Could you check a few things on this model? Use its own coordinates, in mm. Face numbers are marked on the shaded views. A direction names the side the tool comes from. Give positions to 0.01 mm unless a question says otherwise; leave off trailing zeros. Loops run counter-clockwise (first coordinate to the right, second up) from the corner with the lowest first, then second, coordinate; pieces in that order, holes last.
1. Imagine slicing it at A-A (z = 14.5). List the corners of the cut face in (x, y) for me, plus the area to 3 significant figures.
2. Thinking about a two-plate mould opening in Z: for the marked faces 3, 4 and 5, which applies, +Z half, -Z half, draft (parallel to the pull), parting line (faces both ways), or undercut?
3. I need wall thicknesses on line 1 along X through (y, z) = (-11, 15); line 2 along Z through (x, y) = (-6.5, 0.5); line 3 along Z through (x, y) = (23, 0.5). Which ranges of each line are inside material? Lowest first, please.
4. For P1, Ø12, axis at y = 9, z = 8.5, coming from the +X side; P2, Ø4, axis at y = 8.5, z = 6.5, coming from the +X side; P3, Ø1, axis at x = -16.5, y = 8, coming from the +Z side, each with a flat end and sliding along its axis, tell me the tip position at first contact or that it passes through.
5. For the marked faces 1 and 2, which set-ups out of +Z, -Z, +X, -X, +Y, -Y let a thin tool reach every point of the face, with its end or its side?
6. Imagine slicing it at C-C (x = 0.5). List the corners of the cut face in (y, z) for me, plus the area to 3 significant figures.
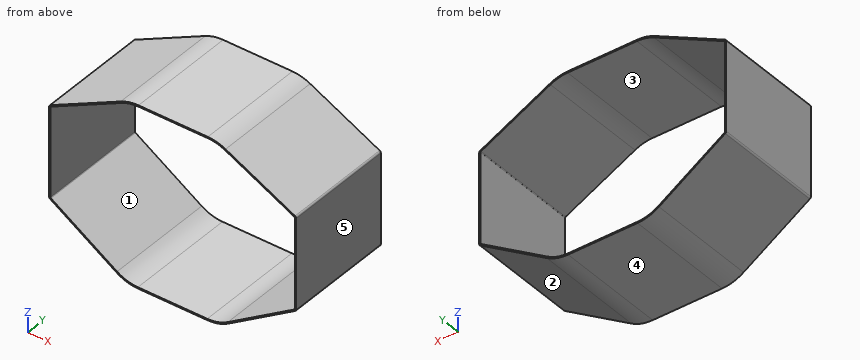
```python
from build123d import *

# Parameters (mm, degrees)
F1_DEPTH = 12.5


with BuildPart() as f1:
    # F0 (on Front) → F1 (new body, symmetric)
    with BuildSketch(Plane.XZ):
        with BuildLine():
            ThreePointArc((-12.775239, 2.986369), (-10.443709, 1.920714), (-7.906317, 1.555622))
            Line((-7.906317, 1.555622), (7.817851, 1.555622))
            ThreePointArc((7.817851, 1.555622), (10.332984, 1.914204), (12.647699, 2.961377))
            Line((12.647699, 2.961377), (27.744712, 12.562894))
            ThreePointArc((27.744712, 12.562894), (27.914658, 12.744133), (27.976387, 12.984796))
            Line((27.976387, 12.984796), (27.976387, 33.317433))
            ThreePointArc((27.976387, 33.317433), (27.901601, 33.580479), (27.699614, 33.764836))
            Line((27.699614, 33.764836), (11.960489, 41.6177))
            ThreePointArc((11.960489, 41.6177), (10.006461, 42.324558), (7.942404, 42.56444))
            Line((7.942404, 42.56444), (-7.7593, 42.56444))
            ThreePointArc((-7.7593, 42.56444), (-9.829371, 42.323139), (-11.78844, 41.612175))
            Line((-11.78844, 41.612175), (-27.736375, 33.627757))
            ThreePointArc((-27.736375, 33.627757), (-27.937928, 33.443415), (-28.012534, 33.180661))
            Line((-28.012534, 33.180661), (-28.012534, 13.060643))
            ThreePointArc((-28.012534, 13.060643), (-27.951423, 12.82111), (-27.783029, 12.640129))
            Line((-27.783029, 12.640129), (-12.775239, 2.986369))
        make_face()
        with BuildLine():
            Line((-12.612941, 3.238677), (-27.620732, 12.892438))
            ThreePointArc((-27.620732, 12.892438), (-27.688089, 12.96483), (-27.712534, 13.060643))
            Line((-27.712534, 13.060643), (-27.712534, 33.180661))
            ThreePointArc((-27.712534, 33.180661), (-27.682691, 33.285763), (-27.60207, 33.3595))
            Line((-27.60207, 33.3595), (-11.654136, 41.343917))
            ThreePointArc((-11.654136, 41.343917), (-9.760369, 42.031183), (-7.7593, 42.26444))
            Line((-7.7593, 42.26444), (7.942404, 42.26444))
            ThreePointArc((7.942404, 42.26444), (9.937659, 42.032554), (11.826553, 41.349258))
            Line((11.826553, 41.349258), (27.565678, 33.496394))
            ThreePointArc((27.565678, 33.496394), (27.646473, 33.422652), (27.676387, 33.317433))
            Line((27.676387, 33.317433), (27.676387, 12.984796))
            ThreePointArc((27.676387, 12.984796), (27.651695, 12.888531), (27.583717, 12.816035))
            Line((27.583717, 12.816035), (12.486704, 3.214518))
            ThreePointArc((12.486704, 3.214518), (10.249146, 2.202252), (7.817851, 1.855622))
            Line((7.817851, 1.855622), (-7.906317, 1.855622))
            ThreePointArc((-7.906317, 1.855622), (-10.359129, 2.208544), (-12.612941, 3.238677))
        make_face(mode=Mode.SUBTRACT)
    extrude(amount=F1_DEPTH, both=True)


solid = f1.part
```
Derived:
1. outline: (-28.01, -12.5) - (-27.71, -12.5) - (-27.71, 12.5) - (-28.01, 12.5) - close; (27.68, -12.5) - (27.98, -12.5) - (27.98, 12.5) - (27.68, 12.5) - close
1. area: 15.0 mm2
2. face 3: undercut
2. face 4: -Z half
2. face 5: draft
3. line 1: x = -28.01 to -27.71, 27.68 to 27.98
3. line 2: z = 1.56 to 1.86, 42.26 to 42.56
3. line 3: z = 9.55 to 9.9, 35.77 to 36.11
4. P1: stops at x = 27.98
4. P2: stops at x = 21.36
4. P3: stops at z = 39.5
5. face 1: +Y, -Y
5. face 2: -Z, +X, +Y, -Y
6. outline: (-12.5, 1.56) - (12.5, 1.56) - (12.5, 1.86) - (-12.5, 1.86) - close; (-12.5, 42.26) - (12.5, 42.26) - (12.5, 42.56) - (-12.5, 42.56) - close
6. area: 15.0 mm2
